Geometry check sheet. Reference: the model listing, model coordinates, mm. Face numbers are marked on the shaded views. Round coordinates to 2 decimals unless told otherwise and drop trailing zeros. Loops run counter-clockwise (first coordinate to the right, second up) from the corner with the lowest first, then second, coordinate; pieces in that order, holes last. Notation, with made-up numbers: M -27.5,47 L 24.5,47 A17 cw 24.5,68 Z; hole C -30,57.5 d10. An arc over 180 degrees is marked long. Write item = value, one per line.
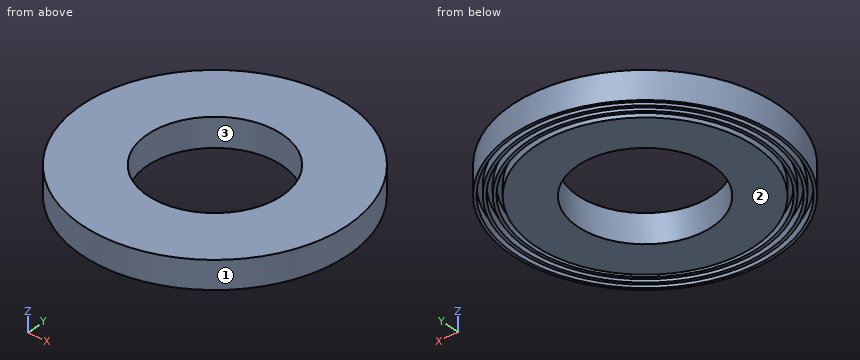
Autodesk Inventor part; units mm, degrees
ref_plane "YZ Plane" through (0, 0, 0) normal (1, 0, 0) x (0, 1, 0)
ref_plane "XZ Plane" through (0, 0, 0) normal (0, 1, 0) x (-1, 0, 0)
ref_plane "XY Plane" through (0, 0, 0) normal (0, 0, 1) x (1, 0, 0)
sketch "Sketch2" plane through (0, 0, 0) normal (0, 0, 1) x (1, 0, 0)
  circle A0 centre (0, 0) radius 70
  circle A1 centre (0, 0) radius 138
  dimension "d1" = 140
  dimension "d2" = 276
extrude "Extrusion1" add sketch "Sketch2" along normal blind 30
sketch "Sketch5" plane through (0, 0, 0) normal (1, 0, 0) x (0, 1, 0)
  line L0 (-138, 0) -> (138, 0)
  line L1 (72.7156, 0) -> (114.2156, 0)
  line L2 (114.2156, 0) -> (114.2156, 11)
  line L3 (114.2156, 11) -> (119.2156, 11)
  line L4 (119.2156, 11) -> (119.2156, 1)
  line L5 (119.2156, 1) -> (122.2156, 1)
  line L6 (122.2156, 1) -> (122.2156, 11)
  line L7 (122.2156, 11) -> (127.2156, 11)
  line L8 (127.2156, 11) -> (127.2156, 1)
  line L9 (127.2156, 1) -> (130.2156, 1)
  line L10 (130.2156, 1) -> (130.2156, 11)
  line L11 (130.2156, 11) -> (135.2156, 11)
  line L12 (135.2156, 11) -> (135.2156, 1)
  line L13 (135.2156, 1) -> (138, 1)
  line L14 (138, 0) -> (138, 30)
  line L15 (0, -6) -> (0, 36)
  point P0 (0, 0)
  dimension "d31" = 41.5
  dimension "d32" = 11
  dimension "d33" = 23.7844
  dimension "d34" = 5
  dimension "d35" = 10
  dimension "d36" = 3
  dimension "d37" = 10
  dimension "d38" = 5
  dimension "d39" = 10
  dimension "d40" = 3
  dimension "d41" = 10
  dimension "d42" = 5
  dimension "d43" = 10
revolve "Revolution3" cut sketch "Sketch5" angle 360 about axis through (0, 0, -10) along (0, 0, 1)
properties part number "lavirinthos_exodos"
(1) Release check for a two-part mould opening along X. For the marked faces 1, 2 and 3 record: released by +X, released by -X, zero draft, split by the parting line, or undercut.
Result set:
face_1 = split by the parting line
face_2 = zero draft
face_3 = undercut
(2) Sectioned sample at C-C on z = 18.75. Record the cut outline in (x, y), then the cut area to 3 significant figures.
Result set:
outline = C 0,0 d276; hole C 0,0 d140
area = 44,400 mm2
(3) Sectioned sample at D-D on y = 81. Record the cut outline in (x, z), then the cut area to 3 significant figures.
Result set:
outline = M -111.73,1 L -108.27,1 L -108.27,11 L -101.96,11 L -101.96,1 L -98.1,1 L -98.1,11 L -91.52,11 L -91.52,1 L -87.47,1 L -87.47,11 L -80.52,11 L -80.52,0 L 80.52,0 L 80.52,11 L 87.47,11 L 87.47,1 L 91.52,1 L 91.52,11 L 98.1,11 L 98.1,1 L 101.96,1 L 101.96,11 L 108.27,11 L 108.27,1 L 111.73,1 L 111.73,30 L -111.73,30 Z
area = 6,240 mm2
(4) Material ranges on line 1 along Y through (x, z) = (0, 19.75); line 2 along Y through (x, z) = (13, 26.25); line 3 along Z through (x, y) = (94.5, 93), recorded low to high. Write a range as from..to.
Result set:
line_1 = -138..-70, 70..138
line_2 = -137.39..-68.78, 68.78..137.39
line_3 = 11..30
(5) Depth check by flat-ended pin: pin 1 Ø3 at (x, z) = (-56.5, 4) entering from +Y; pin 2 Ø4 at (x, z) = (-108.5, 12) entering from +Y; pin 3 Ø4 at (x, z) = (18.5, 17) entering from -Y. Enter the tip coordinate at first touch or a pass-through.
Result set:
pin_1 = 126.57
pin_2 = 87.76
pin_3 = -137.01
